from build123d import *

# Parameters (mm, degrees)
ESQUISSE1_W                        = 30
ESQUISSE1_H                        = 30
BOSS_EXTRU_1_DEPTH                 = 2
BOSS_EXTRU_5_DEPTH                 = 10
CONG_1_R                           = 1
ESQUISSE2_R                        = 3.6
BOSS_EXTRU_6_DEPTH                 = 5
R_P_TITION_CIRCULAIRE1_COUNT       = 3
R_P_TITION_CIRCULAIRE1_ANGLE       = 180
CONG_1_OF_R_P_TITION_CIRCULAIRE1_R = 1
CONG_2_R                           = 2
CONG_3_R                           = 1
CONG_4_R                           = 2


with BuildPart() as part:
    # Esquisse1 → Boss.-Extru.1 (new body)
    with BuildSketch(Plane.XY):
        with Locations((15, 15)):
            Rectangle(ESQUISSE1_W, ESQUISSE1_H)
    extrude(amount=BOSS_EXTRU_1_DEPTH)

    # Esquisse5 → Boss.-Extru.5 (add)
    with BuildSketch(Plane.XY.offset(2)):
        Polygon((27.7, 6.4), (27.7, 23.6), (25.05, 23.6), (21.6, 19.2), (21.6, 10.8), (25.05, 6.4), align=None)
    boss_extru_5 = extrude(amount=BOSS_EXTRU_5_DEPTH)

    # Congé1
    cong_1_edges = [part.edges().sort_by_distance(p)[0] for p in [
        (25.05, 6.4, 7),
        (27.7, 6.4, 7),
        (27.7, 23.6, 7),
        (25.05, 23.6, 7),
        (21.6, 19.2, 7),
        (21.6, 10.8, 7),
    ]]
    fillet(cong_1_edges, radius=CONG_1_R)

    # Esquisse2 → Boss.-Extru.6 (add)
    with BuildSketch(Plane.XY.offset(2)):
        with Locations(Location((15, 15, 0), (0, 0, 180))):
            Circle(ESQUISSE2_R)
    extrude(amount=BOSS_EXTRU_6_DEPTH)

    # Répétition circulaire1: Boss.-Extru.5 ×3 about axis
    r_p_tition_circulaire1_axis = Axis((15, 15, 0), (0, 0, 1))
    for i in range(1, R_P_TITION_CIRCULAIRE1_COUNT):
        add(boss_extru_5.rotate(r_p_tition_circulaire1_axis, i * R_P_TITION_CIRCULAIRE1_ANGLE / (R_P_TITION_CIRCULAIRE1_COUNT - 1)))

    # Congé1 of Répétition circulaire1
    cong_1_of_r_p_tition_circulaire1_edges = [part.edges().sort_by_distance(p)[0] for p in [
        (23.6, 25.05, 7),
        (23.6, 27.7, 7),
        (6.4, 27.7, 7),
        (6.4, 25.05, 7),
        (10.8, 21.6, 7),
        (19.2, 21.6, 7),
        (4.95, 23.6, 7),
        (2.3, 23.6, 7),
        (2.3, 6.4, 7),
        (4.95, 6.4, 7),
        (8.4, 10.8, 7),
        (8.4, 19.2, 7),
    ]]
    fillet(cong_1_of_r_p_tition_circulaire1_edges, radius=CONG_1_OF_R_P_TITION_CIRCULAIRE1_R)

    # Congé2
    cong_2_edges = [part.edges().sort_by_distance(p)[0] for p in [
        (0, 30, 1),
        (30, 30, 1),
        (30, 0, 1),
        (0, 0, 1),
    ]]
    fillet(cong_2_edges, radius=CONG_2_R)

    # Congé3
    cong_3_edges = [part.edges().sort_by_distance(p)[0] for p in [
        (15, 27.7, 12),
        (23.6, 26.118328167, 12),
        (6.4, 26.118328167, 12),
        (8.655619048, 23.28138961, 12),
        (15, 21.6, 12),
        (21.344380952, 23.28138961, 12),
        (6.500824998, 25.099067124, 12),
        (10.818910387, 21.654764961, 12),
        (19.181089613, 21.654764961, 12),
        (23.499175002, 25.099067124, 12),
        (6.692893219, 27.407106781, 12),
        (23.307106781, 27.407106781, 12),
        (2.3, 15, 12),
        (3.881671833, 23.6, 12),
        (3.881671833, 6.4, 12),
        (6.71861039, 8.655619048, 12),
        (8.4, 15, 12),
        (6.71861039, 21.344380952, 12),
        (4.900932876, 6.500824998, 12),
        (8.345235039, 10.818910387, 12),
        (8.345235039, 19.181089613, 12),
        (4.900932876, 23.499175002, 12),
        (2.592893219, 6.692893219, 12),
        (2.592893219, 23.307106781, 12),
        (27.7, 15, 12),
        (26.118328167, 6.4, 12),
        (26.118328167, 23.6, 12),
        (23.28138961, 21.344380952, 12),
        (21.6, 15, 12),
        (23.28138961, 8.655619048, 12),
        (25.099067124, 23.499175002, 12),
        (21.654764961, 19.181089613, 12),
        (21.654764961, 10.818910387, 12),
        (25.099067124, 6.500824998, 12),
        (27.407106781, 23.307106781, 12),
        (27.407106781, 6.692893219, 12),
        (18.6, 15, 7),
    ]]
    fillet(cong_3_edges, radius=CONG_3_R)

    # Congé4
    cong_4_edges = [part.edges().sort_by_distance(p)[0] for p in [
        (29.414213562, 29.414213562, 0),
        (15, 30, 0),
        (0.585786438, 29.414213562, 0),
        (0, 15, 0),
        (0.585786438, 0.585786438, 0),
        (15, 0, 0),
        (29.414213562, 0.585786438, 0),
        (30, 15, 0),
    ]]
    fillet(cong_4_edges, radius=CONG_4_R - 0.0001)  # a hair under: the kernel refuses the full size


solid = part.part
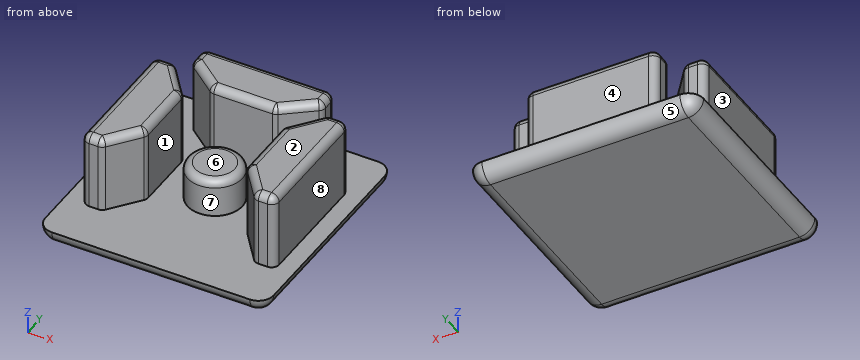
Model file for the job. Use its own axes, mm. Face numbers are marked on the shaded views. A direction names the side the tool comes from. Round coordinates to 2 decimals unless told otherwise and drop trailing zeros. Write each question's results on one line, items separated by ' | '. Start each with the question number.
(1) Probe probe 1 along X at (y, z) = (8.25, 7); probe 2 along X at (y, z) = (17.5, 8.5); probe 3 along Y at (x, z) = (11.5, 8.5). List the from-to ranges inside material, lowest first. Write a range as from..to.
(2) Drop flat-ended pins along their axis: pin 1 (6 mm diameter, centred on y = 20, z = 9.5, fed in from +X); pin 2 (0.6 mm diameter, centred on x = 3.5, z = 5, fed in from +Y); pin 3 (5 mm diameter, centred on x = 26, z = 9, fed in from -Y). Give the stop position or say it passes through.
(3) Saw through at C-C, the plane z = 5.25. State how many separate pieces and enclosed holes the cut face has, then the cut area to 3 significant figures.
(4) Which spindle directions (+Z, -Z, +X, -X, +Y, -Y) get a long thin tool onto all of the face, cutting with end or side? Do the marked faces 4, 5, 6, 7 and 8. Say none if no direction does.
(5) Two-plate mould, pull along X, no slides. Class the marked faces 1, 2 and 3: pulls with the +X half, pulls with the -X half, needs draft (parallel to the pull), parting line crosses it, or undercut.
Established:
1) probe 1: x = 2.3..6.4, 23.6..27.7 | probe 2: x = 2.3..8.4, 21.6..27.7 | probe 3: y = 21.6..27.7
2) pin 1: stops at x = 27.7 | pin 2: stops at y = 23.6 | pin 3: stops at y = 6.4
3) separate pieces: 4 | enclosed holes: 0 | area: 308 mm^2
4) face 4: +Z, +X, -X, +Y | face 5: -Z, +X, -X, +Y | face 6: +Z, -Y | face 7: +Z | face 8: +Z, +X, +Y, -Y
5) face 1: undercut | face 2: needs draft | face 3: pulls with the -X half
